Geometry: final body of the model. Coordinates: model frame, mm. A direction names the side the tool comes from. Coordinates: 2 decimals unless noted, no trailing zeros. Loops run counter-clockwise (first coordinate to the right, second up) from the corner with the lowest first, then second, coordinate; pieces in that order, holes last. Notation, with made-up numbers: (49.5, -21) - (55.5, -21) arc R21 ccw to (55.5, 7) - close; hole circle Ø3 at (46.5, 77). An arc over 180 degrees is marked (long way). Put each result on its own line as item: value. Start each with the question number.
1) Section A-A on z = 14. Output: boundary loops of the cut face in (x, y), and give its area (3 significant figures).
2) Reachability of faces 4 (the flat face through (1.5, 0.7, 8)), 5 (the flat face through (2.6, 1.5, 13.9)), 6 (the cylindrical face through (0.748, 0.976, 15.69)) from +Z, -Z, +X, -X, +Y, -Y: full face, straight path, thin tool, end or side. Return the list, or none.
3) Material intervals for line 1 along Y through (x, z) = (0, 16.75); line 2 along X through (y, z) = (-0.8, 18.5); line 3 along Y through (x, z) = (0.5, 15), sorted ascending. Write a range as from..to.
4) Contact query for flat-ended pins moving along their axis: pin 1 Ø2 at (y, z) = (-2, 6) entering from +X; pin 2 Ø1 at (y, z) = (1.5, 7) entering from -X; pin 3 Ø3 at (y, z) = (-0.5, 2) entering from -X (3 decimals). Output: stop coordinate, or through.
5) Section B-B on z = 2.75. Output: boundary loops of the cut face in (x, y) (3 decimals).
6) Draft query along X for faces 1 (the flat face through (2.6, -1.5, 13.9)), 2 (the conical face through (-0.21, 0.05, 10.89)), 3 (the flat face through (0, 3, 14)). Return one class per face: +X half, -X half, draft (parallel to the pull), parting line (faces both ways), or undercut.
7) Section D-D on y = -2.2. Output: boundary loops of the cut face in (x, z), and give its area (3 significant figures).
8) Section C-C on x = -2. Output: boundary loops of the cut face in (y, z).
Autodesk Inventor part; units mm, degrees
ref_plane "Plan YZ" through (0, 0, 0) normal (1, 0, 0) x (0, 1, 0)
ref_plane "Plan XZ" through (0, 0, 0) normal (0, 1, 0) x (-1, 0, 0)
ref_plane "Plan XY" through (0, 0, 0) normal (0, 0, 1) x (1, 0, 0)
sketch "Esquisse1" plane through (0, 0, 0) normal (0, 0, 1) x (1, 0, 0)
  circle A0 centre (0, 0) radius 1.425
  dimension "d0" = 2.85
extrude "Extrusion1" add sketch "Esquisse1" along normal blind 8
sketch "Esquisse6" plane through (0, 0, 8) normal (0, 0, 1) x (1, 0, 0)
  line L0 (-4.8497, 0) -> (4.8497, 0) construction
  line L1 (0, -4.2) -> (0, 4.2) construction
  line L2 (-1.7321, -3) -> (-3.4641, 0)
  line L3 (-3.4641, 0) -> (-1.7321, 3)
  line L4 (-1.7321, 3) -> (0, 3)
  line L5 (-1.7321, -3) -> (0, -3)
  line L6 (1.7321, -3) -> (3.4641, 0)
  line L7 (3.4641, 0) -> (1.7321, 3)
  line L8 (1.7321, 3) -> (0, 3)
  line L9 (1.7321, -3) -> (0, -3)
  point P0 (0, 0)
  dimension "d4" = 6
  dimension "d8" = 120
  dimension "d10" = 6
extrude "Extrusion2" add sketch "Esquisse6" along normal blind 12
sketch "Esquisse7" plane through (0, 0, 20) normal (0, 0, 1) x (1, 0, 0)
  circle A0 centre (0, 0) radius 1.425
hole "Perçage1" at (0, 0, 20) direction (0, 0, -1) diameter 2.459 depth 8.5 tip angle 118
thread "Filetage1"
properties part number "entretoise12xM3" material "."
Answer block:
1. outline: (-3.46, 0) - (-1.73, -3) - (1.73, -3) - (3.46, 0) - (1.73, 3) - (-1.73, 3) - close; hole circle Ø2.46 at (0, 0)
1. area: 26.4 mm²
2. face 4: -Z
2. face 5: +Z, -Z, +X, +Y
2. face 6: +Z
3. line 1: y = -3..-1.23, 1.23..3
3. line 2: x = -3..-0.93, 0.93..3
3. line 3: y = -3..-1.12, 1.12..3
4. pin 1: stops at x = 1.02
4. pin 2: stops at x = -1.02
4. pin 3: stops at x = -1.425
5. outline: circle Ø2.85 at (0, 0)
6. face 1: +X half
6. face 2: undercut
6. face 3: draft
7. outline: (-2.19, 8) - (2.19, 8) - (2.19, 20) - (-2.19, 20) - close
7. area: 52.7 mm²
8. outline: (-2.54, 8) - (2.54, 8) - (2.54, 20) - (-2.54, 20) - close
